Part model, mm, in its own coordinate system. Coordinates: 2 decimals unless noted, no trailing zeros. Loops run counter-clockwise (first coordinate to the right, second up) from the corner with the lowest first, then second, coordinate; pieces in that order, holes last. Notation, with made-up numbers: (49, 79) -> (75, 79) arc R23 cw to (75, 101) -> close; hole circle Ø5 at (64, -3.5). An arc over 180 degrees is marked (long way). Use one line per item in the form item = value. Start each with the question number.
(1) Band-saw the part on B-B on y = 245.5. Give the cut face in (x, z), then the cut area to 3 significant figures.
(2) Drill centre lines: L1, parallel to Y at x = 143, z = 2; L2, parallel to Y at x = 66.5, z = 5.5; L3, parallel to X at y = 198, z = 7.75. Where is each one in solid material? Low to high. Write a range as [from, to].
(3) Band-saw the part on A-A on x = 73.5. Give the cut face in (y, z), then the cut area to 3 significant figures.
(4) Pin check, flat tips, straight feed: P1, Ø1.5, axis at y = 123, z = 6, coming from the -X side; P2, Ø1.1, axis at x = 153, z = 2.5, coming from the +Y side; P3, Ø1, axis at x = 151.5, z = 5, coming from the -Y side. Stop position of each tip, or through.
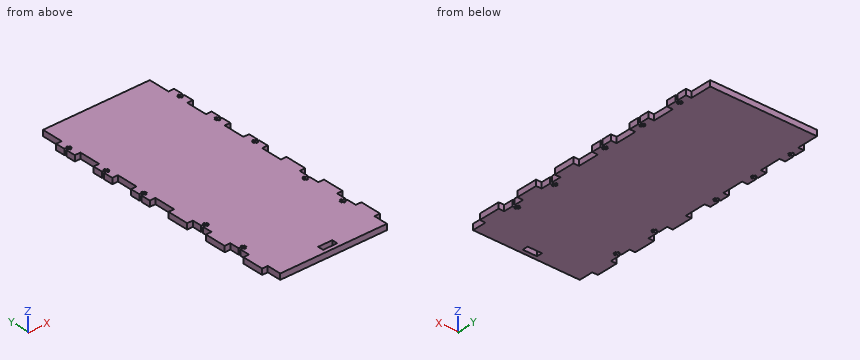
```python
from build123d import *

# Parameters (mm, degrees)
SKETCH1_W           = 150
SKETCH1_H           = 380
SKETCH1_W_2         = 20
SKETCH1_H_2         = 8
BOSS_EXTRUDE1_DEPTH = 8
SKETCH2_W           = 7.9
SKETCH2_H           = 30
BOSS_EXTRUDE2_DEPTH = 8
CUT_EXTRUDE2_DEPTH  = 9


with BuildPart() as part:
    # Sketch1 → Boss-Extrude1 (new body)
    with BuildSketch(Plane.XY):
        with Locations((75, 190)):
            Rectangle(SKETCH1_W, SKETCH1_H)
        with Locations((75, 9.5)):
            Rectangle(SKETCH1_W_2, SKETCH1_H_2, mode=Mode.SUBTRACT)
    extrude(amount=BOSS_EXTRUDE1_DEPTH)

    # Sketch2 → Boss-Extrude2 (add)
    with BuildSketch(Plane.XY.offset(8)):
        with Locations((153.95, 335)):
            Rectangle(SKETCH2_W, SKETCH2_H)
        with Locations((-3.95, 335)):
            Rectangle(SKETCH2_W, SKETCH2_H)
        with Locations((153.95, 275)):
            Rectangle(SKETCH2_W, SKETCH2_H)
        with Locations((-3.95, 275)):
            Rectangle(SKETCH2_W, SKETCH2_H)
        with Locations((153.95, 215)):
            Rectangle(SKETCH2_W, SKETCH2_H)
        with Locations((-3.95, 215)):
            Rectangle(SKETCH2_W, SKETCH2_H)
        with Locations((153.95, 155)):
            Rectangle(SKETCH2_W, SKETCH2_H)
        with Locations((-3.95, 155)):
            Rectangle(SKETCH2_W, SKETCH2_H)
        with Locations((153.95, 95)):
            Rectangle(SKETCH2_W, SKETCH2_H)
        with Locations((-3.95, 95)):
            Rectangle(SKETCH2_W, SKETCH2_H)
        with Locations((153.95, 35)):
            Rectangle(SKETCH2_W, SKETCH2_H)
        with Locations((-3.95, 35)):
            Rectangle(SKETCH2_W, SKETCH2_H)
    extrude(amount=-BOSS_EXTRUDE2_DEPTH)

    # Sketch3 → Cut-Extrude2 (cut, through all)
    with BuildSketch(Plane(origin=(0, 0, 0), x_dir=(-1, 0, 0), z_dir=(0, 0, -1))):
        Polygon((7.9, 273.35), (7.9, 276.65), (4.3, 276.65), (4.3, 278.5), (2.1, 278.5), (2.1, 276.65), (0.1, 276.65), (0.1, 273.35), (2.1, 273.35), (2.1, 271.5), (4.3, 271.5), (4.3, 273.35), align=None)
        Polygon((7.9, 333.35), (7.9, 336.65), (4.3, 336.65), (4.3, 338.5), (2.1, 338.5), (2.1, 336.65), (0.1, 336.65), (0.1, 333.35), (2.1, 333.35), (2.1, 331.5), (4.3, 331.5), (4.3, 333.35), align=None)
        Polygon((7.9, 213.35), (7.9, 216.65), (4.3, 216.65), (4.3, 218.5), (2.1, 218.5), (2.1, 216.65), (0.1, 216.65), (0.1, 213.35), (2.1, 213.35), (2.1, 211.5), (4.3, 211.5), (4.3, 213.35), align=None)
        Polygon((-157.9, 213.35), (-154.3, 213.35), (-154.3, 211.5), (-152.1, 211.5), (-152.1, 213.35), (-150.1, 213.35), (-150.1, 216.65), (-152.1, 216.65), (-152.1, 218.5), (-154.3, 218.5), (-154.3, 216.65), (-157.9, 216.65), align=None)
        Polygon((-157.9, 273.35), (-154.3, 273.35), (-154.3, 271.5), (-152.1, 271.5), (-152.1, 273.35), (-150.1, 273.35), (-150.1, 276.65), (-152.1, 276.65), (-152.1, 278.5), (-154.3, 278.5), (-154.3, 276.65), (-157.9, 276.65), align=None)
        Polygon((-157.9, 333.35), (-154.3, 333.35), (-154.3, 331.5), (-152.1, 331.5), (-152.1, 333.35), (-150.1, 333.35), (-150.1, 336.65), (-152.1, 336.65), (-152.1, 338.5), (-154.3, 338.5), (-154.3, 336.65), (-157.9, 336.65), align=None)
        Polygon((0, 123.35), (0, 126.65), (-4, 126.65), (-4, 128.5), (-6.2, 128.5), (-6.2, 126.65), (-8.2, 126.65), (-8.2, 123.35), (-6.2, 123.35), (-6.2, 121.5), (-4, 121.5), (-4, 123.35), align=None)
        Polygon((0, 63.35), (0, 66.65), (-4, 66.65), (-4, 68.5), (-6.2, 68.5), (-6.2, 66.65), (-8.2, 66.65), (-8.2, 63.35), (-6.2, 63.35), (-6.2, 61.5), (-4, 61.5), (-4, 63.35), align=None)
        Polygon((-150, 63.35), (-146, 63.35), (-146, 61.5), (-143.8, 61.5), (-143.8, 63.35), (-141.8, 63.35), (-141.8, 66.65), (-143.8, 66.65), (-143.8, 68.5), (-146, 68.5), (-146, 66.65), (-150, 66.65), align=None)
        Polygon((-150, 123.35), (-146, 123.35), (-146, 121.5), (-143.8, 121.5), (-143.8, 123.35), (-141.8, 123.35), (-141.8, 126.65), (-143.8, 126.65), (-143.8, 128.5), (-146, 128.5), (-146, 126.65), (-150, 126.65), align=None)
    extrude(amount=-CUT_EXTRUDE2_DEPTH, mode=Mode.SUBTRACT)


solid = part.part
```
A:
q1.outline = (0, 0) -> (150, 0) -> (150, 8) -> (0, 8) -> close
q1.area = 1,200 mm²
q2.L1 = [0, 63.35], [66.65, 123.35], [126.65, 380]
q2.L2 = [0, 5.5], [13.5, 380]
q2.L3 = [0, 150]
q3.outline = (0, 0) -> (5.5, 0) -> (5.5, 8) -> (0, 8) -> close; (13.5, 0) -> (380, 0) -> (380, 8) -> (13.5, 8) -> close
q3.area = 2,980 mm²
q4.P1 = 0
q4.P2 = 350
q4.P3 = 20
